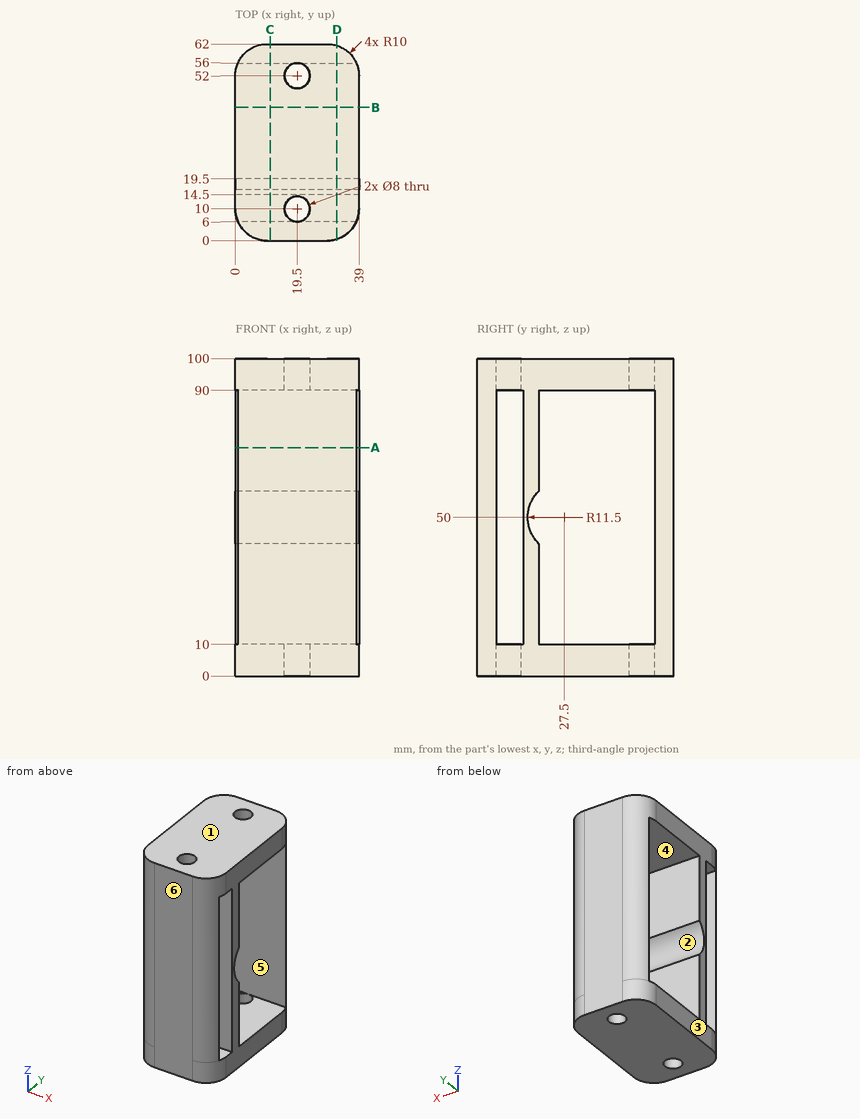
The figure shows three views and two pictorial views of one solid part (mm, origin at its lowest corner). Answer the questions. A direction names the side the tool comes from. Give positions to 0.01 mm unless a question says otherwise; leave off trailing zeros. Order: outer loops, then holes, each group sorted by start corner. A loop starts at its lowest first (then second) coordinate and runs counter-clockwise, first axis right, second up. Notation, with made-up numbers: (2, 29.25) -> (30, 29.25) arc R19 cw to (30, 62.25) -> close; hole circle Ø10 at (-32, 15). An arc over 180 degrees is marked (long way). One line per item, written item: value.
1) Find section C-C, the plane x = 11. Determine the outline of the cut face in (y, z).
Reported:
outline: (0, 0) -> (62, 0) -> (62, 100) -> (0, 100) -> close; hole (6, 10) -> (14.5, 10) -> (14.5, 90) -> (6, 90) -> close; hole (19.5, 10) -> (56, 10) -> (56, 90) -> (19.5, 90) -> (19.5, 58.26) arc R11.5 ccw to (19.5, 41.74) -> close
2) Find section B-B, the plane y = 42. Determine the outline of the cut face in (x, z).
Reported:
outline: (0, 0) -> (39, 0) -> (39, 10) -> (0, 10) -> close; (0, 90) -> (39, 90) -> (39, 100) -> (0, 100) -> close
3) Find section D-D, the plane x = 32. Determine the outline of the cut face in (y, z).
Reported:
outline: (0.46, 0) -> (61.54, 0) -> (61.54, 100) -> (0.46, 100) -> close; hole (6, 10) -> (14.5, 10) -> (14.5, 90) -> (6, 90) -> close; hole (19.5, 10) -> (56, 10) -> (56, 90) -> (19.5, 90) -> (19.5, 58.26) arc R11.5 ccw to (19.5, 41.74) -> close
4) Determine the mould class of the marked faces 3, 4, 5 and 6 for opening direction Y: pulls with the +Y half, pulls with the -Y half, needs draft (parallel to the pull), parting line crosses it, or undercut.
Reported:
face 3: needs draft
face 4: undercut
face 5: undercut
face 6: pulls with the -Y half
5) Find the intervals of material crossed by line 1 (Y direction, x = 27.5, z = 73); line 2 (Z direction, x = 7, y = 44.5); line 3 (X direction, y = 10, z = 94.5), in increasing order.
Reported:
line 1: y = 0 to 6, 14.5 to 19.5, 56 to 62
line 2: z = 0 to 10, 90 to 100
line 3: x = 0 to 15.5, 23.5 to 39
6) A tool of negligible diameter and unlimited length cuts with its end or side. For the marked faces 1 and 2, from which of +Z, -Z, +X, -X, +Y, -Y can it reach the whole face along a straight path? Write none if from no direction.
Reported:
face 1: +Z, +X, -X, +Y, -Y
face 2: +X, -X
7) A flat-ended cylindrical pin translates along its axis: P1, Ø2, axis at x = 6, z = 24, coming from the +Y side. Find the tip coordinate at first contact, or state that the pin passes through.
Reported:
P1: stops at y = 61.54
8) Find section A-A, the plane z = 72. Determine the outline of the cut face in (x, y).
Reported:
outline: (0, 14.5) -> (39, 14.5) -> (39, 19.5) -> (0, 19.5) -> close; (0.83, 6) arc R10 ccw to (10, 0) -> (29, 0) arc R10 ccw to (38.17, 6) -> close; (0.83, 56) -> (38.17, 56) arc R10 ccw to (29, 62) -> (10, 62) arc R10 ccw to start
